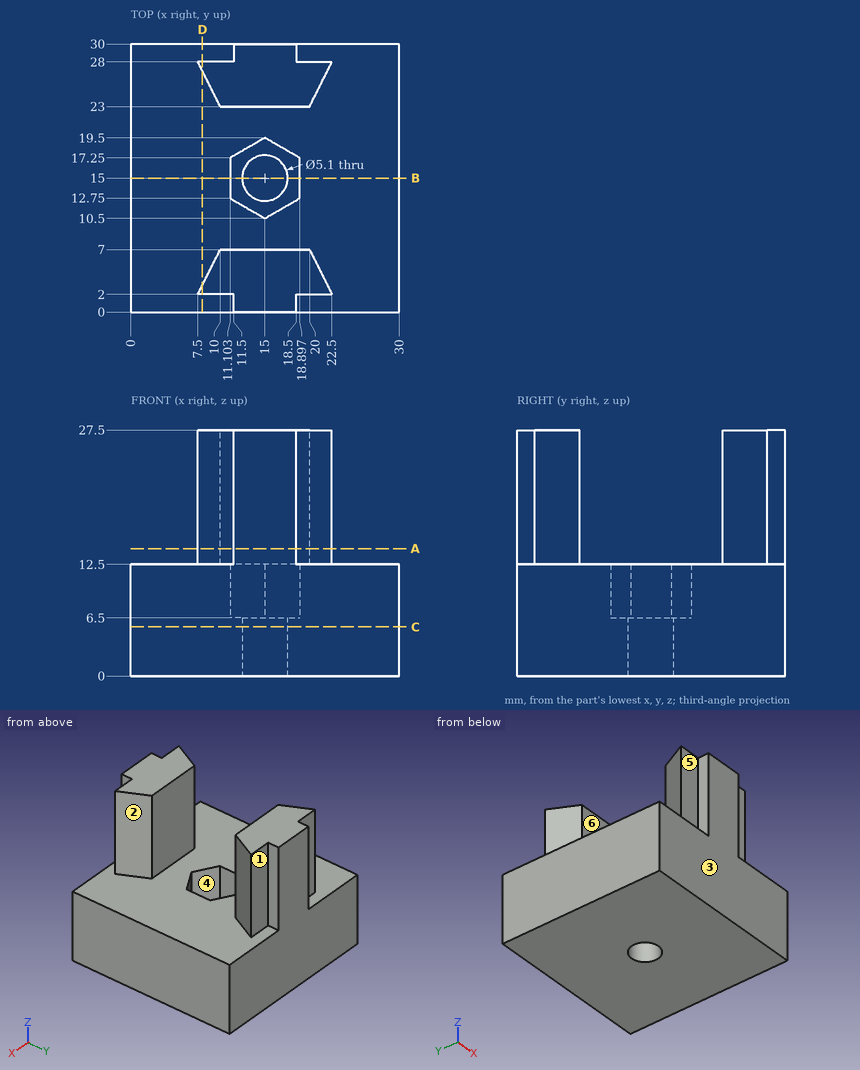
Geometry check sheet. Reference: drawing and pictorial views, mm from the part's lowest x, y, z. A direction names the side the tool comes from. Give positions to 0.01 mm unless a question says otherwise; leave off trailing zeros. Order: outer loops, then holes, each group sorted by start corner. A loop starts at its lowest first (then second) coordinate and runs counter-clockwise, first axis right, second up. Notation, with made-up numbers: (6, 60.25) - (13, 60.25) arc R27 ccw to (13, 82.25) - close; hole circle Ø6 at (-30.5, 78.25). An arc over 180 degrees is marked (long way). Answer as CSV lines item,"result".
1. Section check C-C (z = 5.5). Record the boundary of the cut face in (x, y).
Result sheet:
outline,"(0, 0) - (30, 0) - (30, 30) - (0, 30) - close; hole circle Ø5.1 at (15, 15)"
2. Go/stop test with flat-tipped pins: P1, Ø2, axis at y = 4, z = 14.5, coming from the -X side; P2, Ø1.6, axis at y = 1.5, z = 23.5, coming from the -X side; P3, Ø8, axis at x = 15, y = 15, coming from the +Z side. Record where each tip stops, or that it passes through.
Result sheet:
P1,"x = 8"
P2,"x = 7.5"
P3,"z = 12.5"
3. Tool access check on the marked faces 4, 5 and 6. Record the directions out of +Z, -Z, +X, -X, +Y, -Y that give a thin tool (end or side, any length) a straight path to the whole face; none if there is none.
Result sheet:
face 4,"+Z"
face 5,"+Z, -X, -Y"
face 6,"+Z, +X, -X"
4. Scan lines: probe 1 along X at (y, z) = (15.75, 6.75); probe 2 along Y at (x, z) = (15, 4). Record each from-to range of solid material in increasing order. Write a range as from..to.
Result sheet:
probe 1,"0..11.1, 18.9..30"
probe 2,"0..12.45, 17.55..30"
5. Section check A-A (z = 14.25). Record the boundary of the cut face in (x, y).
Result sheet:
outline,"(7.5, 2) - (11.5, 2) - (11.5, 0) - (18.5, 0) - (18.5, 2) - (22.5, 2) - (20, 7) - (10, 7) - close; (7.5, 28) - (10, 23) - (20, 23) - (22.5, 28) - (18.5, 28) - (18.5, 30) - (11.5, 30) - (11.5, 28) - close"
6. Section check B-B (y = 15). Record the boundary of the cut face in (x, z), then the cut area to 3 significant figures.
Result sheet:
outline,"(0, 0) - (12.45, 0) - (12.45, 6.5) - (11.1, 6.5) - (11.1, 12.5) - (0, 12.5) - close; (17.55, 0) - (30, 0) - (30, 12.5) - (18.9, 12.5) - (18.9, 6.5) - (17.55, 6.5) - close"
area,"295 mm²"
7. Mould release check, pull along Y, two halves, no side actions. Record for the marked faces 1, 2 and 3: released by +Y, released by -Y, zero draft, split by the parting line, or undercut.
Result sheet:
face 1,"released by +Y"
face 2,"undercut"
face 3,"released by -Y"
8. Section check D-D (x = 8). Record the boundary of the cut face in (y, z).
Result sheet:
outline,"(0, 0) - (30, 0) - (30, 12.5) - (28, 12.5) - (28, 27.5) - (27, 27.5) - (27, 12.5) - (3, 12.5) - (3, 27.5) - (2, 27.5) - (2, 12.5) - (0, 12.5) - close"
